from build123d import *

# Parameters (mm, degrees)
SKETCH_1_W      = 10
SKETCH_1_H      = 40
SKETCH_1_R      = 2.1
EXTRUDE_1_DEPTH = 30
FILLET_1_R      = 3


with BuildPart() as part:
    # 草图1 → 凸台-拉伸1 (new body)
    with BuildSketch(Plane(origin=(0, 0, 0), x_dir=(1, 0, 0), z_dir=(0, 1, 0))):
        with Locations((-5, -20)):
            Rectangle(SKETCH_1_W, SKETCH_1_H)
        with Locations((-5, -7)):
            Circle(SKETCH_1_R, mode=Mode.SUBTRACT)
        with Locations((-5, -33)):
            Circle(SKETCH_1_R, mode=Mode.SUBTRACT)
    extrude(amount=EXTRUDE_1_DEPTH)

    # 圆角1
    fillet_1_edges = [part.edges().sort_by_distance(p)[0] for p in [
        (-10, 15, 0),
        (0, 15, 0),
        (0, 15, 40),
        (-10, 15, 40),
    ]]
    fillet(fillet_1_edges, radius=FILLET_1_R)


solid = part.part
Could you check a few things on this model? Use its own coordinates, in mm. Coordinates: 2 decimals unless noted, no trailing zeros. Order: outer loops, then holes, each group sorted by start corner. A loop starts at its lowest first (then second) coordinate and runs counter-clockwise, first axis right, second up. Notation, with made-up numbers: (-3, 88.25) -> (32, 88.25) arc R10 ccw to (32, 95.25) -> close; hole circle Ø11 at (79, -1). An arc over 180 degrees is marked (long way). One line per item, written item: value. Start each with the question number.
1) If I drill on L1, parallel to Z at x = -5, y = 16.75; L2, parallel to X at y = 20.25, z = 33; L3, parallel to Z at x = -4.5, y = 6, over which ranges is the centre line in solid material (lowest first)? Write a range as [from, to].
2) Imagine slicing it at A-A on x = -5. List the corners of the cut face in (y, z) for me, plus the area to 3 significant figures.
3) Imagine slicing it at B-B on y = 7.25. List the corners of the cut face in (x, z) for me.
4) Imagine slicing it at C-C on z = 33. List the corners of the cut face in (x, y) for me, plus the area to 3 significant figures.
5) Imagine slicing it at D-D on x = -1. List the corners of the cut face in (y, z) for me.
6) We'd pull the mould along X, two halves only. Please class faces 1 (the flat face through (-5, 30, 20)), 2 (the flat face through (-10, 15, 20)), 3 (the cylindrical face through (-5.273, 14.79, 4.918)): +X half, -X half, draft (parallel to the pull), parting line (faces both ways), or undercut.
7) I'm going to push a flat-ended pin straight in: pin 1 (2.5 mm diameter, centred on x = -5, z = 7, fed in from -Y). Where does the tip first touch, or does it pass through?
Answer list:
1. L1: z = [0, 4.9], [9.1, 30.9], [35.1, 40]
1. L2: x = [-10, -7.1], [-2.9, 0]
1. L3: z = [0, 4.96], [9.04, 30.96], [35.04, 40]
2. outline: (0, 0) -> (30, 0) -> (30, 4.9) -> (0, 4.9) -> close; (0, 9.1) -> (30, 9.1) -> (30, 30.9) -> (0, 30.9) -> close; (0, 35.1) -> (30, 35.1) -> (30, 40) -> (0, 40) -> close
2. area: 948 mm2
3. outline: (-10, 3) arc R3 ccw to (-7, 0) -> (-3, 0) arc R3 ccw to (0, 3) -> (0, 37) arc R3 ccw to (-3, 40) -> (-7, 40) arc R3 ccw to (-10, 37) -> close; hole circle Ø4.2 at (-5, 7); hole circle Ø4.2 at (-5, 33)
4. outline: (-10, 0) -> (-7.1, 0) -> (-7.1, 30) -> (-10, 30) -> close; (-2.9, 0) -> (0, 0) -> (0, 30) -> (-2.9, 30) -> close
4. area: 174 mm2
5. outline: (0, 0.76) -> (30, 0.76) -> (30, 39.24) -> (0, 39.24) -> close
6. face 1: draft
6. face 2: -X half
6. face 3: undercut
7. pin 1: passes through
